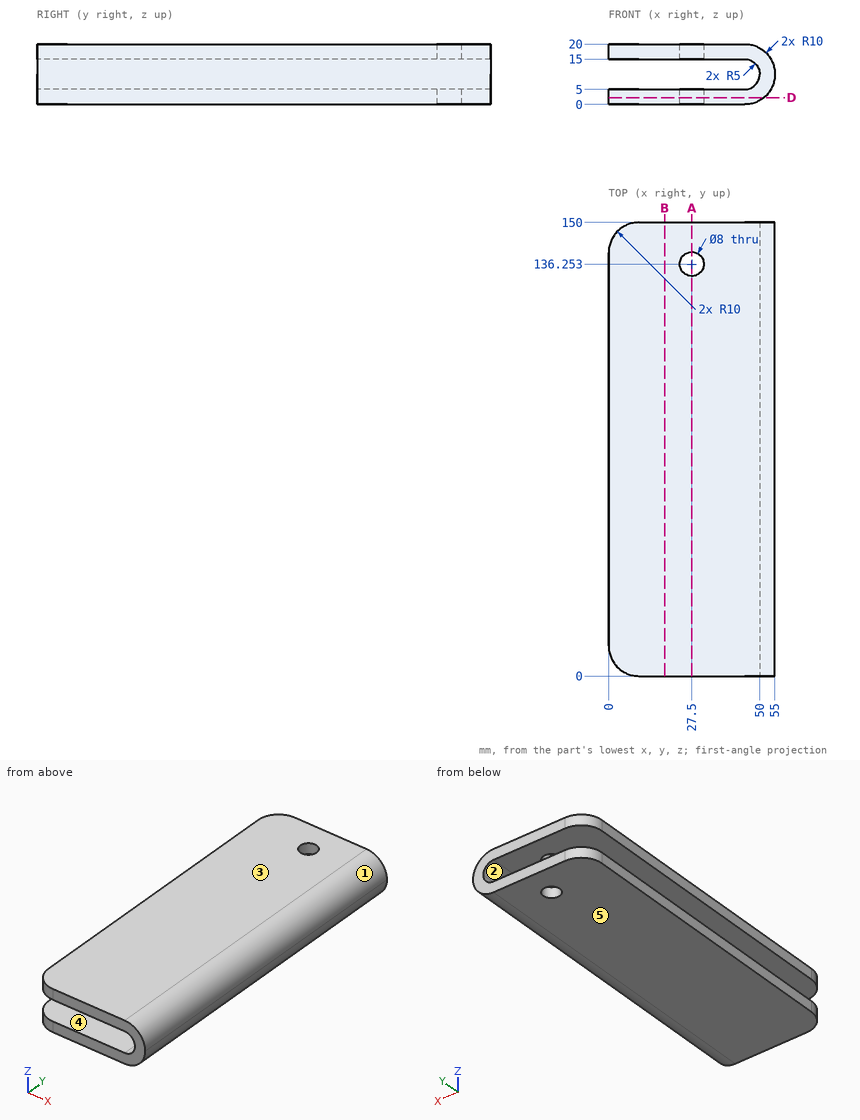
Source: three-view drawing plus pictorial views. Frame: mm from the lowest corner of the part. A direction names the side the tool comes from. Round coordinates to 2 decimals unless told otherwise and drop trailing zeros. Loops run counter-clockwise (first coordinate to the right, second up) from the corner with the lowest first, then second, coordinate; pieces in that order, holes last.
1. Mould query, pull axis Z, two halves, no side actions, for the marked faces 3, 4 and 5. Classes: released by +Z, released by -Z, zero draft, split by the parting line, or undercut.
2. Contact query for flat-ended pins moving along their axis: pin 1 (4 mm diameter, centred on y = 106.5, z = 15, fed in from -X); pin 2 (10 mm diameter, centred on y = 129.5, z = 3.5, fed in from +X); pin 3 (2 mm diameter, centred on y = 66, z = 5, fed in from +X) (1 decimal). Output: stop coordinate, or through.
3. Ray query, L1, parallel to Z at x = 32.5, y = 112.5; L2, parallel to Y at x = 27.5, z = 19; L3, parallel to Z at x = 48, y = 19. Return the intervals inside material, ascending.
4. Access query for the marked faces 1 and 2. Directions: +Z, -Z, +X, -X, +Y, -Y. A direction counts if a zero-diameter tool reaches every point of the face in a straight line with its end or side. Return the directions, or none.
5. Section query D-D on z = 2.25. Output: boundary loops of the cut face in (x, y).
6. Section query A-A on x = 27.5. Output: boundary loops of the cut face in (y, z).
7. Section query B-B on x = 18.5. Output: boundary loops of the cut face in (y, z).
Answers below:
1. face 3: released by +Z
1. face 4: undercut
1. face 5: released by -Z
2. pin 1: stops at x = 0
2. pin 2: stops at x = 54.89
2. pin 3: stops at x = 54.2
3. L1: z = 0 to 5, 15 to 20
3. L2: y = 0 to 132.25, 140.25 to 150
3. L3: z = 0.46 to 6, 14 to 19.54
4. face 1: +Z, +X, +Y, -Y
4. face 2: -X, +Y, -Y
5. outline: (0, 10) arc R10 ccw to (10, 0) - (51.32, 0) - (51.32, 150) - (10, 150) arc R10 ccw to (0, 140) - close; hole circle Ø8 at (27.5, 136.25)
6. outline: (0, 0) - (132.25, 0) - (132.25, 5) - (0, 5) - close; (0, 15) - (132.25, 15) - (132.25, 20) - (0, 20) - close; (140.25, 0) - (150, 0) - (150, 5) - (140.25, 5) - close; (140.25, 15) - (150, 15) - (150, 20) - (140.25, 20) - close
7. outline: (0, 0) - (150, 0) - (150, 5) - (0, 5) - close; (0, 15) - (150, 15) - (150, 20) - (0, 20) - close
